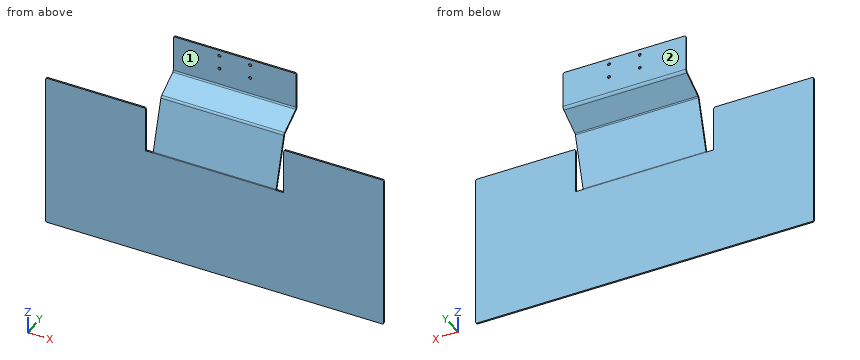
from build123d import *

# Parameters (mm, degrees)
BASE_FLANGE1_DEPTH           = 203.2
SKETCH2_W                    = 196.85
SKETCH2_H                    = 181.790367069
BOSS_EXTRUDE1_DEPTH          = 2.58826
F_10_0_1935_DIAMETER_HOLE1_D = 4.9149
SKETCH16_W                   = 184.15
SKETCH16_H                   = 76.2
BOSS_EXTRUDE2_DEPTH          = 2.58826
SKETCH17_W                   = 19.05
SKETCH17_H                   = 257.990367069
CUT_EXTRUDE1_DEPTH           = 537.279077243
FILLET1_R                    = 2.54


# Sheet-metal steps are written as plain solids
with BuildPart() as part:
    # Sketch1 → Base-Flange1 (new body)
    with BuildSketch(Plane(origin=(0, 0, 0), x_dir=(0, 0, -1), z_dir=(1, 0, 0))):
        with BuildLine():
            Line((0, 0), (-181.790367069, 0))
            ThreePointArc((-181.790367069, 0), (-182.617352358, 0.059641748), (-183.427221345, 0.237332575))
            Line((-183.427221345, 0.237332575), (-265.029897441, 24.40914646))
            ThreePointArc((-265.029897441, 24.40914646), (-266.980756871, 25.424699599), (-268.409129334, 27.097108878))
            Line((-268.409129334, 27.097108878), (-288.093120118, 61.888444803))
            ThreePointArc((-288.093120118, 61.888444803), (-289.257017075, 63.067677729), (-290.856499452, 63.5))
            Line((-290.856499452, 63.5), (-350.980894178, 63.5))
            Line((-350.980894178, 63.5), (-350.980894178, 66.08826))
            Line((-350.980894178, 66.08826), (-290.856499452, 66.08826))
            ThreePointArc((-290.856499452, 66.08826), (-287.953119041, 65.303508614), (-285.840413284, 63.162965007))
            Line((-285.840413284, 63.162965007), (-266.156422501, 28.371629081))
            ThreePointArc((-266.156422501, 28.371629081), (-265.369527137, 27.450292987), (-264.294791885, 26.890821227))
            Line((-264.294791885, 26.890821227), (-182.692115789, 2.719007342))
            ThreePointArc((-182.692115789, 2.719007342), (-182.245956144, 2.621116847), (-181.790367069, 2.58826))
            Line((-181.790367069, 2.58826), (0, 2.58826))
            Line((0, 2.58826), (0, 0))
        make_face()
    extrude(amount=BASE_FLANGE1_DEPTH)

    # Sketch2 → Boss-Extrude1 (add)
    with BuildSketch(Plane(origin=(0, 2.58826, 0), x_dir=(1, 0, 0), z_dir=(0, 1, 0))):
        with Locations((-98.425, -90.895183535)):
            Rectangle(SKETCH2_W, SKETCH2_H)
        with Locations((301.625, -90.895183535)):
            Rectangle(SKETCH2_W, SKETCH2_H)
    extrude(amount=-BOSS_EXTRUDE1_DEPTH)

    # #10 (0.1935) Diameter Hole1 (through all)
    with Locations(Plane(origin=(0, 66.08826, 0), x_dir=(1, 0, 0), z_dir=(0, 1, 0))):
        with Locations((76.2, -341.455894178), (76.2, -318.646694178), (127, -318.646694178), (127, -341.455894178)):
            Hole(F_10_0_1935_DIAMETER_HOLE1_D / 2)

    # Sketch16 → Boss-Extrude2 (add)
    with BuildSketch(Plane(origin=(0, 2.58826, 0), x_dir=(1, 0, 0), z_dir=(0, 1, 0))):
        with Locations((-104.775, -219.890367069)):
            Rectangle(SKETCH16_W, SKETCH16_H)
        with Locations((307.975, -219.890367069)):
            Rectangle(SKETCH16_W, SKETCH16_H)
    extrude(amount=-BOSS_EXTRUDE2_DEPTH)

    # Sketch17 → Cut-Extrude1 (cut, through all)
    with BuildSketch(Plane.XZ):
        with Locations((-187.325, 128.995183535)):
            Rectangle(SKETCH17_W, SKETCH17_H)
        with Locations((390.525, 128.995183535)):
            Rectangle(SKETCH17_W, SKETCH17_H)
    extrude(amount=-CUT_EXTRUDE1_DEPTH, mode=Mode.SUBTRACT)

    # Fillet1
    fillet1_edges = [part.edges().sort_by_distance(p)[0] for p in [
        (-12.7, 1.29413, 257.990367069),
        (215.9, 1.29413, 257.990367069),
        (381, 1.29413, 257.990367069),
        (-177.8, 1.29413, 257.990367069),
        (-177.8, 1.29413, 0),
        (381, 1.29413, 0),
        (0, 64.79413, 350.980894178),
        (203.2, 64.79413, 350.980894178),
    ]]
    fillet(fillet1_edges, radius=FILLET1_R)


solid = part.part
Could you check a few things on this model? Use its own coordinates, in mm. Face numbers are marked on the shaded views. A direction names the side the tool comes from. Give positions to 0.01 mm unless a question says otherwise; leave off trailing zeros. Write each loop counter-clockwise with the first axis right and the second up, starting at its lowest first coordinate (ties: lowest second). Pieces come first, ordered by that corner, then holes. Notation, with made-up numbers: (79.25, 20) -> (123.25, 20) arc R20 ccw to (123.25, 38) -> close; hole circle Ø1 at (48, -40). An arc over 180 degrees is marked (long way). Answer as CSV lines item,"result". Start each with the question number.
(1) If we section it at C-C, the plane y = 10: Write out the boundary of the cut face in (x, z).
(2) If we section it at B-B, the plane z = 32.5: Write out the boundary of the cut face in (x, y), and give its area (3 significant figures).
(3) Which directions (+Z, -Z, +X, -X, +Y, -Y) give clear straight access to the entire face, cutting with the end or side of a thin tool? Please do the marked faces 1 and 2.
(4) Please list where these lines run through material, in increasing order: line 1 (Z direction, x = 76, y = 64); line 2 (Z direction, x = 76.2, y = 65.2); line 3 (Y direction, x = 309, z = 249.5).
(5) I'm going to push flat-ended pins straight in: pin 1 Ø2 at (x, y) = (-8.5, 2) entering from +Z; pin 2 Ø18 at (x, z) = (76.5, 307.5) entering from -Y; pin 3 Ø10 at (x, z) = (118.5, 253) entering from -Y. Where does each tip first touch, or does it pass through?
Answer list:
1,outline,"(0, 207.27) -> (203.2, 207.27) -> (203.2, 216.39) -> (0, 216.39) -> close"
2,outline,"(-177.8, 0) -> (381, 0) -> (381, 2.59) -> (-177.8, 2.59) -> close"
2,area,"1,450 mm^2"
3,face 1,"+Z, +X, -X, -Y"
3,face 2,"+Z, -Z, +X, -X, +Y"
4,line 1,"286.42 to 316.2, 321.1 to 339.01, 343.91 to 350.98"
4,line 2,"287.78 to 316.19, 321.1 to 339, 343.91 to 350.98"
4,line 3,"0 to 2.59"
5,pin 1,"z = 181.79"
5,pin 2,"y = 63.5"
5,pin 3,"y = 19.36"
